The figure shows three views and two pictorial views of one solid part (mm, origin at its lowest corner). Answer the questions. A direction names the side the tool comes from. Coordinates: 2 decimals unless noted, no trailing zeros. Loops run counter-clockwise (first coordinate to the right, second up) from the corner with the lowest first, then second, coordinate; pieces in that order, holes last.
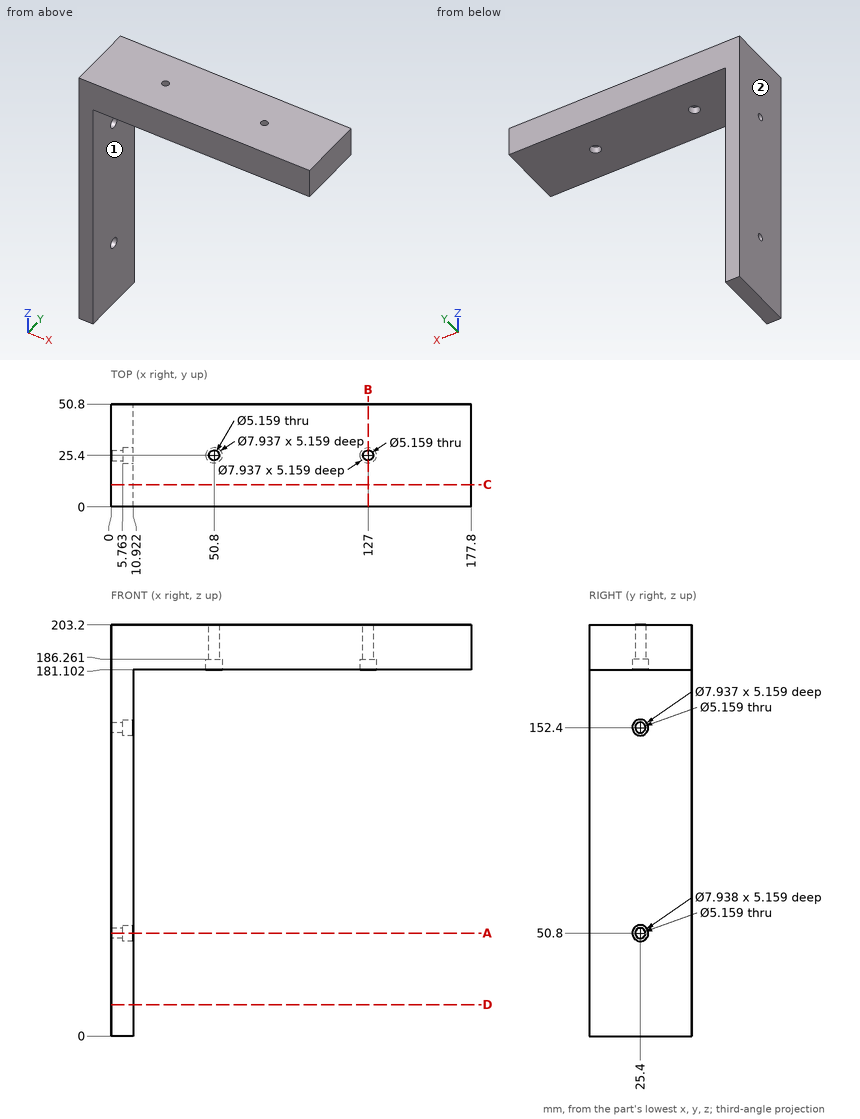
1. A cutting plane is placed at C-C, the plane y = 11. Give the vertices of the cut face in (x, z).
2. A cutting plane is placed at B-B, the plane x = 127. Give the vertices of the cut face in (y, z), then the cut area to 3 significant figures.
3. Straight lines are drawn through the part: probe 1 along Z at (x, y) = (7, 25); probe 2 along Y at (x, z) = (7.05, 50.8); probe 3 along Y at (x, z) = (2.1, 152.4). For each, find the intervals that lie inside material, in ascending order.
4. For the marked faces 1 and 2, determine the directions among +Z, -Z, +X, -X, +Y, -Y from which every point of the face is accessible in a straight line to the end or side of a thin tool.
5. Each of these flat-tipped pins is pushed along its axis until it touches: P1, Ø3, axis at y = 25.4, z = 152.4, coming from the -X side (3 decimals); P2, Ø4, axis at x = 49.5, y = 26, coming from the -Z side; P3, Ø8.5, axis at y = 26.5, z = 51, coming from the +X side; P4, Ø6.5, axis at x = 128, y = 26, coming from the -Z side. Where does it stop, or does it pass through?
6. A cutting plane is placed at D-D, the plane z = 15.5. Give the vertices of the cut face in (x, y), then the cut area to 3 significant figures.
7. A cutting plane is placed at A-A, the plane z = 50.8. Give the vertices of the cut face in (x, y).
Answers below:
1. outline: (0, 0) - (10.92, 0) - (10.92, 181.1) - (177.8, 181.1) - (177.8, 203.2) - (0, 203.2) - close
2. outline: (0, 181.1) - (21.43, 181.1) - (21.43, 186.26) - (22.82, 186.26) - (22.82, 203.2) - (0, 203.2) - close; (27.98, 186.26) - (29.37, 186.26) - (29.37, 181.1) - (50.8, 181.1) - (50.8, 203.2) - (27.98, 203.2) - close
2. area: 994 mm2
3. probe 1: z = 0 to 46.85, 54.75 to 148.45, 156.35 to 203.2
3. probe 2: y = 0 to 21.43, 29.37 to 50.8
3. probe 3: y = 0 to 22.82, 27.98 to 50.8
4. face 1: -Z, +X, +Y, -Y
4. face 2: +Z, -Z, -X, +Y, -Y
5. P1: passes through
5. P2: stops at z = 186.26
5. P3: stops at x = 10.92
5. P4: stops at z = 181.1
6. outline: (0, 0) - (10.92, 0) - (10.92, 50.8) - (0, 50.8) - close
6. area: 555 mm2
7. outline: (0, 0) - (10.92, 0) - (10.92, 21.43) - (5.76, 21.43) - (5.76, 22.82) - (0, 22.82) - close; (0, 27.98) - (5.76, 27.98) - (5.76, 29.37) - (10.92, 29.37) - (10.92, 50.8) - (0, 50.8) - close
